Input: part model. Units: mm. Frame: model coordinates. A direction names the side the tool comes from. Coordinates: 2 decimals unless noted, no trailing zeros. One line per question, with ' | ' between items.
from build123d import *

# Parameters (mm, degrees)
F0_W      = 58
F0_H      = 46
F1_DEPTH  = 6
F2_W      = 11
F2_H      = 7
F3_DEPTH  = 6.001
F4_W      = 13
F4_H      = 9
F4_W_2    = 11
F4_H_2    = 7
F5_DEPTH  = 5
F6_W      = 6
F6_H      = 6
F7_DEPTH  = 4
F8_W      = 6
F8_H      = 6
F9_DEPTH  = 4
F10_R     = 0.75
F11_DEPTH = 6.001


with BuildPart() as f1:
    # F0 (on Top) → F1 (new body)
    with BuildSketch(Plane.XY):
        Rectangle(F0_W, F0_H)
    extrude(amount=F1_DEPTH)

    # F2 (on face) → F3 (cut, through all)
    with BuildSketch(Plane.XY.offset(6)):
        with Locations((-21, 16.5)):
            Rectangle(F2_W, F2_H)
        with Locations((-7, 16.5)):
            Rectangle(F2_W, F2_H)
        with Locations((7, 16.5)):
            Rectangle(F2_W, F2_H)
        with Locations((21, 16.5)):
            Rectangle(F2_W, F2_H)
        with Locations((-20.923837, 5.500264)):
            Rectangle(F2_W, F2_H)
        with Locations((-6.923837, 5.500264)):
            Rectangle(F2_W, F2_H)
        with Locations((7.076163, 5.500264)):
            Rectangle(F2_W, F2_H)
        with Locations((21.076163, 5.500264)):
            Rectangle(F2_W, F2_H)
        with Locations((-20.847673, -5.499473)):
            Rectangle(F2_W, F2_H)
        with Locations((-6.847673, -5.499473)):
            Rectangle(F2_W, F2_H)
        with Locations((7.152327, -5.499473)):
            Rectangle(F2_W, F2_H)
        with Locations((21.152327, -5.499473)):
            Rectangle(F2_W, F2_H)
        with Locations((-20.77151, -16.499209)):
            Rectangle(F2_W, F2_H)
        with Locations((-6.77151, -16.499209)):
            Rectangle(F2_W, F2_H)
        with Locations((7.22849, -16.499209)):
            Rectangle(F2_W, F2_H)
        with Locations((21.22849, -16.499209)):
            Rectangle(F2_W, F2_H)
    extrude(amount=-F3_DEPTH, mode=Mode.SUBTRACT)

    # F4 (on face) → F5 (cut)
    with BuildSketch(Plane.XY.offset(6)):
        with Locations((-21, 16.5)):
            Rectangle(F4_W, F4_H)
        with Locations((-21, 16.5)):
            Rectangle(F4_W_2, F4_H_2, mode=Mode.SUBTRACT)
        with Locations((-7, 16.5)):
            Rectangle(F4_W, F4_H)
        with Locations((-7, 16.5)):
            Rectangle(F4_W_2, F4_H_2, mode=Mode.SUBTRACT)
        with Locations((7, 16.5)):
            Rectangle(F4_W, F4_H)
        with Locations((7, 16.5)):
            Rectangle(F4_W_2, F4_H_2, mode=Mode.SUBTRACT)
        with Locations((21, 16.5)):
            Rectangle(F4_W, F4_H)
        with Locations((21, 16.5)):
            Rectangle(F4_W_2, F4_H_2, mode=Mode.SUBTRACT)
        with Locations((-21, 5.5)):
            Rectangle(F4_W, F4_H)
        with Locations((-20.923837, 5.500264)):
            Rectangle(F4_W_2, F4_H_2, mode=Mode.SUBTRACT)
        with Locations((7, 5.5)):
            Rectangle(F4_W, F4_H)
        with Locations((7.076163, 5.500264)):
            Rectangle(F4_W_2, F4_H_2, mode=Mode.SUBTRACT)
        with Locations((-7, 5.5)):
            Rectangle(F4_W, F4_H)
        with Locations((-6.923837, 5.500264)):
            Rectangle(F4_W_2, F4_H_2, mode=Mode.SUBTRACT)
        with Locations((21, 5.5)):
            Rectangle(F4_W, F4_H)
        with Locations((21.076163, 5.500264)):
            Rectangle(F4_W_2, F4_H_2, mode=Mode.SUBTRACT)
        with Locations((-21, -5.5)):
            Rectangle(F4_W, F4_H)
        with Locations((-20.847673, -5.499473)):
            Rectangle(F4_W_2, F4_H_2, mode=Mode.SUBTRACT)
        with Locations((-7, -5.5)):
            Rectangle(F4_W, F4_H)
        with Locations((-6.847673, -5.499473)):
            Rectangle(F4_W_2, F4_H_2, mode=Mode.SUBTRACT)
        with Locations((7, -5.5)):
            Rectangle(F4_W, F4_H)
        with Locations((7.152327, -5.499473)):
            Rectangle(F4_W_2, F4_H_2, mode=Mode.SUBTRACT)
        with Locations((21, -5.5)):
            Rectangle(F4_W, F4_H)
        with Locations((21.152327, -5.499473)):
            Rectangle(F4_W_2, F4_H_2, mode=Mode.SUBTRACT)
        with Locations((-21, -16.5)):
            Rectangle(F4_W, F4_H)
        with Locations((-20.77151, -16.499209)):
            Rectangle(F4_W_2, F4_H_2, mode=Mode.SUBTRACT)
        with Locations((-7, -16.5)):
            Rectangle(F4_W, F4_H)
        with Locations((-6.77151, -16.499209)):
            Rectangle(F4_W_2, F4_H_2, mode=Mode.SUBTRACT)
        with Locations((7, -16.5)):
            Rectangle(F4_W, F4_H)
        with Locations((7.22849, -16.499209)):
            Rectangle(F4_W_2, F4_H_2, mode=Mode.SUBTRACT)
        with Locations((21, -16.5)):
            Rectangle(F4_W, F4_H)
        with Locations((21.22849, -16.499209)):
            Rectangle(F4_W_2, F4_H_2, mode=Mode.SUBTRACT)
    extrude(amount=-F5_DEPTH, mode=Mode.SUBTRACT)

    # F6 (on face) → F7 (join)
    with BuildSketch(Plane.XZ.offset(23)):
        with Locations((19, 3)):
            Rectangle(F6_W, F6_H)
        with Locations((-19, 3)):
            Rectangle(F6_W, F6_H)
    extrude(amount=F7_DEPTH)

    # F8 (on face) → F9 (join)
    with BuildSketch(Plane(origin=(0, 23, 0), x_dir=(-1, 0, 0), z_dir=(0, 1, 0))):
        with Locations((19, 3)):
            Rectangle(F8_W, F8_H)
        with Locations((-19, 3)):
            Rectangle(F8_W, F8_H)
    extrude(amount=F9_DEPTH)

    # F10 (on face) → F11 (cut, through all)
    with BuildSketch(Plane.XY.offset(6)):
        with Locations((-19, 24.222791)):
            Circle(F10_R)
    extrude(amount=-F11_DEPTH, mode=Mode.SUBTRACT)


solid = f1.part
Item 1: Draft query along X for faces 4 (the face through (19, -27, 3)), 5 (the face through (-21.1, 12.6, 1)), 6 (the face through (22, -25, 3)). Return one class per face: released by +X, released by -X, zero draft, split by the parting line, or undercut.
Data:
face 4: zero draft | face 5: undercut | face 6: released by +X
Item 2: Access query for faces 1 (the face through (-21, -1, 4)), 2 (the face through (19, 27, 3)), 3 (the face through (-26, -23, 3)). Directions: +Z, -Z, +X, -X, +Y, -Y. A direction counts if a zero-diameter tool reaches every point of the face in a straight line with its end or side. Return the directions, or none.
Data:
face 1: +Z | face 2: +Z, -Z, +X, -X, +Y | face 3: +Z, -Z, -X, -Y
Item 3: Section A-A on y = -16.5. Count the separate pieces of the cut face and the enclosed holes in it, and give its area (3 significant figures).
Data:
separate pieces: 5 | enclosed holes: 0 | area: 44.0 mm^2
Item 4: Contact query for flat-ended pins moving along their axis: P1, Ø4.5, axis at x = 6.5, y = -3.5, coming from the +Z side; P2, Ø0.5, axis at x = 23, z = 0.5, coming from the -Y side; P3, Ø1, axis at x = 5.5, z = 4, coming from the +Y side. Output: stop coordinate, or through.
Data:
P1: z = 1 | P2: y = -23 | P3: y = 23
Item 5: Ray query, line 1 (X direction, y = -15, z = 4.35); line 2 (Y direction, x = -19, z = 2.6); line 3 (Y direction, x = 19, z = 5.05). Return the intervals inside material, ascending.
Data:
line 1: -29 to -27.5, -14.5 to -13.5, -0.5 to 0.5, 13.5 to 14.5, 27.5 to 29 | line 2: -27 to -21, -12 to -10, -1 to 1, 10 to 12, 21 to 23.47, 24.97 to 27 | line 3: -27 to -21, -12 to -10, -1 to 1, 10 to 12, 21 to 27
